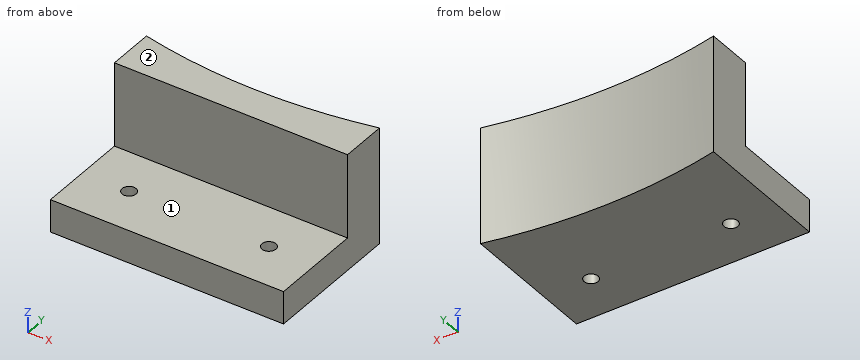
from build123d import *

# Parameters (mm, degrees)
F0_W     = 50
F0_H     = 30
F1_DEPTH = 25
F3_DEPTH = 25
F4_W     = 50
F4_H     = 20
F5_DEPTH = 18
F6_R     = 1.5
F7_DEPTH = 25


with BuildPart() as f1:
    # F0 (on Top) → F1 (new body)
    with BuildSketch(Plane.XY):
        Rectangle(F0_W, F0_H)
    extrude(amount=F1_DEPTH)

    # F2 (on face) → F3 (cut)
    with BuildSketch(Plane.XY.offset(25)):
        with BuildLine():
            Line((25, 15), (-25, 15))
            ThreePointArc((-25, 15), (0, 12.249722), (25, 15))
        make_face()
    extrude(amount=-F3_DEPTH, mode=Mode.SUBTRACT)

    # F4 (on face) → F5 (cut)
    with BuildSketch(Plane.XY.offset(25)):
        with Locations((0, -5)):
            Rectangle(F4_W, F4_H)
    extrude(amount=-F5_DEPTH, mode=Mode.SUBTRACT)

    # F6 (on face) → F7 (cut)
    with BuildSketch(Plane.XY.offset(7)):
        with Locations((-15, -5)):
            Circle(F6_R)
        with Locations((15, -5)):
            Circle(F6_R)
    extrude(amount=-F7_DEPTH, mode=Mode.SUBTRACT)


solid = f1.part
Work out the finished part from the listing and answer in its coordinate system (mm). Face numbers are marked on the shaded views. A direction names the side the tool comes from. Give positions to 0.01 mm unless a question says otherwise; leave off trailing zeros. Write each loop counter-clockwise with the first axis right and the second up, starting at its lowest first coordinate (ties: lowest second). Pieces come first, ordered by that corner, then holes. Notation, with made-up numbers: (-27, 51.5) - (18, 51.5) arc R20 cw to (18, 56.5) - close; hole circle Ø10 at (-27, 80.25). An arc over 180 degrees is marked (long way). One line per item, written item: value. Start each with the question number.
1. Find section C-C (z = 3.5). Write down the section's boundary in (x, y).
2. Find section A-A (y = -5). Write down the section's boundary in (x, z), then the cut area to 3 significant figures.
3. For the marked faces 1 and 2, determine the directions among +Z, -Z, +X, -X, +Y, -Y from which every point of the face is accessible in a straight line to the end or side of a thin tool.
4. Consider probe 1 along X at (y, z) = (-4, 1.75); probe 2 along Z at (x, y) = (-11.5, 0.5); probe 3 along Y at (x, z) = (-15, 3). Determine where each line is inside the solid, lowest interval first.
5. Find section D-D (y = 13.25). Write down the section's boundary in (x, z), then the cut area to 3 significant figures.
6. Given pin 1 (10 mm diameter, centred on x = -5, z = 14.5, fed in from +Y); pin 2 (8 mm diameter, centred on x = 3, y = -3.5, fed in from +Z); pin 3 (1.5 mm diameter, centred on x = -18, z = 18.5, fed in from -Y), each flat-ended and moving along its own axis, determine where each tip first touches the part or whether it passes through.
7. Find section B-B (x = 15). Write down the section's boundary in (y, z), then the cut area to 3 significant figures.
Geometry results:
1. outline: (-25, -15) - (25, -15) - (25, 15) arc R115 cw to (-25, 15) - close; hole circle Ø3 at (-15, -5); hole circle Ø3 at (15, -5)
2. outline: (-25, 0) - (-16.5, 0) - (-16.5, 7) - (-25, 7) - close; (-13.5, 0) - (13.5, 0) - (13.5, 7) - (-13.5, 7) - close; (16.5, 0) - (25, 0) - (25, 7) - (16.5, 7) - close
2. area: 308 mm2
3. face 1: +Z, +X, -X, -Y
3. face 2: +Z, +X, -X, +Y, -Y
4. probe 1: -25 to -16.12, -13.88 to 13.88, 16.12 to 25
4. probe 2: 0 to 7
4. probe 3: -15 to -6.5, -3.5 to 13.23
5. outline: (-25, 0) - (-15.13, 0) - (-15.13, 25) - (-25, 25) - close; (15.13, 0) - (25, 0) - (25, 25) - (15.13, 25) - close
5. area: 493 mm2
6. pin 1: y = 12.69
6. pin 2: z = 7
6. pin 3: y = 5
7. outline: (-15, 0) - (-6.5, 0) - (-6.5, 7) - (-15, 7) - close; (-3.5, 0) - (13.23, 0) - (13.23, 25) - (5, 25) - (5, 7) - (-3.5, 7) - close
7. area: 325 mm2
